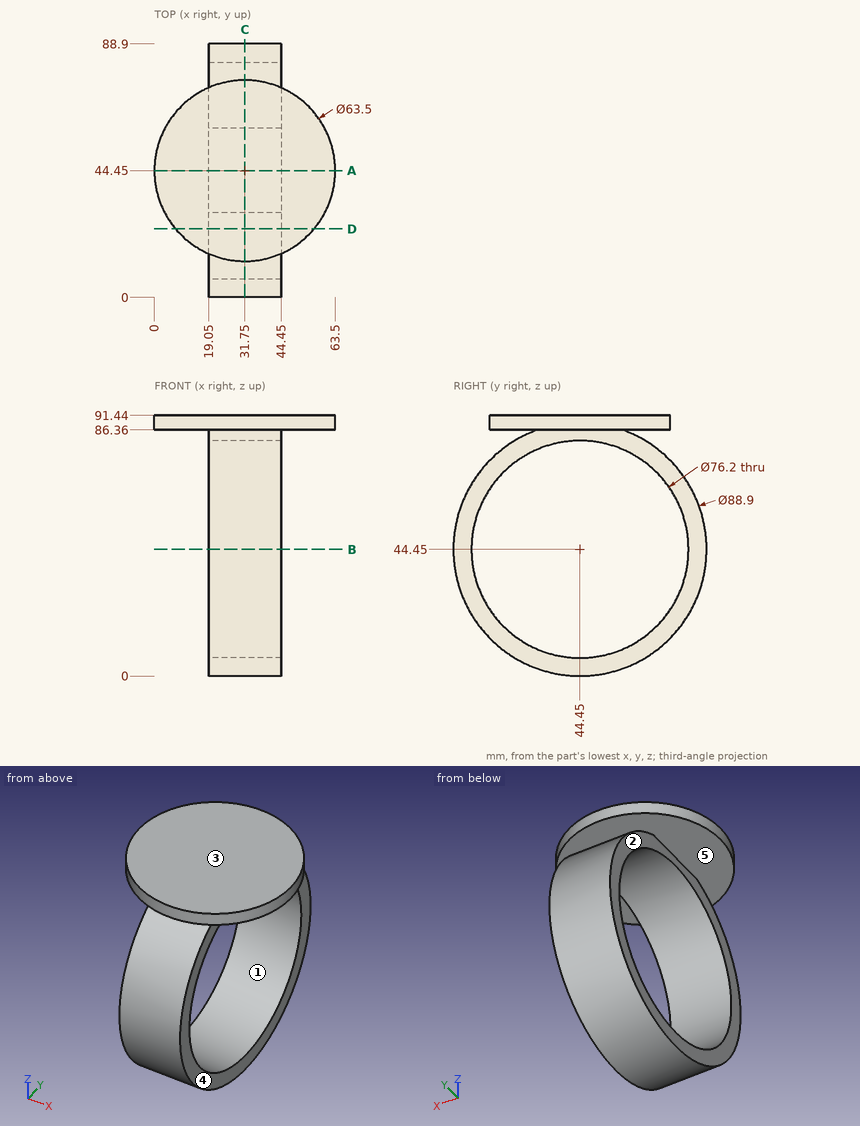
Design review of the part shown in the three views and the two pictorial views. Dimensions are in mm from the part's minimum x, y and z. A direction names the side the tool comes from. Give positions to 0.01 mm unless a question says otherwise; leave off trailing zeros. Write each loop counter-clockwise with the first axis right and the second up, starting at its lowest first coordinate (ties: lowest second). Pieces come first, ordered by that corner, then holes.
Item 1: Take a section at D-D (y = 24). Give the boundary of the cut face in (x, z), and give its area (3 significant figures).
Item 2: Wall thickness on probe 1 along Z at (x, y) = (35.25, 44.45); probe 2 along Y at (x, z) = (31, 44); probe 3 along X at (y, z) = (7.5, 60): over which ranges is each line inside the solid? List them lowest first.
Item 3: Machinability: for the marked faces 1 and 2, which of the approach directions +Z, -Z, +X, -X, +Y, -Y give a long, thin tool a straight path to every point of the face, cutting with its end or side? Answer none if there is none.
Item 4: Insertion check: P1, Ø19, axis at x = 30.5, y = 36, coming from the -Z side; P2, Ø5, axis at y = 43, z = 80.5, coming from the +X side; P3, Ø10, axis at y = 17, z = 29.5, coming from the +X side. Each pin has a flat end and moves straight along its axis. Give the tip position at first contact, or say it passes through.
Item 5: The part is to be moulded in two halves that separate along Z. For the marked faces 3, 4 and 5, say which applies: +Z half, -Z half, draft (parallel to the pull), parting line (faces both ways), or undercut.
Item 6: Take a section at C-C (x = 31.75). Give the boundary of the cut face in (y, z), and give its area (3 significant figures).
Item 7: Take a section at B-B (z = 44.45). Give the boundary of the cut face in (x, y).
Item 8: Take a section at A-A (y = 44.45). Give the boundary of the cut face in (x, z).
Established:
1. outline: (7.46, 86.36) - (56.04, 86.36) - (56.04, 91.44) - (7.46, 91.44) - close; (19.05, 4.98) - (44.45, 4.98) - (44.45, 12.3) - (19.05, 12.3) - close; (19.05, 76.6) - (44.45, 76.6) - (44.45, 83.92) - (19.05, 83.92) - close
1. area: 619 mm2
2. probe 1: z = 0 to 6.35, 82.55 to 91.44
2. probe 2: y = 0 to 6.35, 82.55 to 88.9
2. probe 3: x = 19.05 to 44.45
3. face 1: +X, -X
3. face 2: -Z, -X, +Y, -Y
4. P1: stops at z = 0
4. P2: stops at x = 44.45
4. P3: passes through
5. face 3: +Z half
5. face 4: draft
5. face 5: undercut
6. outline: (12.7, 86.36) - (29.64, 86.36) arc R44.45 ccw (long way) to (59.26, 86.36) - (76.2, 86.36) - (76.2, 91.44) - (12.7, 91.44) - close; hole circle Ø76.2 at (44.45, 44.45)
6. area: 1,920 mm2
7. outline: (19.05, 0) - (44.45, 0) - (44.45, 6.35) - (19.05, 6.35) - close; (19.05, 82.55) - (44.45, 82.55) - (44.45, 88.9) - (19.05, 88.9) - close
8. outline: (0, 86.36) - (19.05, 86.36) - (19.05, 82.55) - (44.45, 82.55) - (44.45, 86.36) - (63.5, 86.36) - (63.5, 91.44) - (0, 91.44) - close; (19.05, 0) - (44.45, 0) - (44.45, 6.35) - (19.05, 6.35) - close
